from build123d import *

# Parameters (mm, degrees)
SKETCH_W        = 30
SKETCH_H        = 25
PAD_DEPTH       = 30
SKETCH001_W     = 20.784298
SKETCH001_H     = 31.024467
POCKET_DEPTH    = 30.001
POCKET001_DEPTH = 104.489578018
SKETCH003_R     = 1.4
POCKET002_DEPTH = 5
CHAMFER_SIZE    = 2
CHAMFER001_SIZE = 2
CHAMFER002_SIZE = 1


with BuildPart() as part:
    # Sketch → Pad (new body)
    with BuildSketch(Plane.XZ):
        with Locations((0, 12.5)):
            Rectangle(SKETCH_W, SKETCH_H)
    extrude(amount=PAD_DEPTH)

    # Sketch001 (on Face2 of Pad) → Pocket (cut, through all)
    with BuildSketch(Plane(origin=(15, 0, 0), x_dir=(0, 0, 1), z_dir=(1, 0, 0))):
        with Locations((16.392149, 19.5122335)):
            Rectangle(SKETCH001_W, SKETCH001_H)
    extrude(amount=-POCKET_DEPTH, mode=Mode.SUBTRACT)

    # Sketch002 (on Face8 of Pocket) → Pocket001 (cut, through all)
    with BuildSketch(Plane(origin=(0, 0, 6), x_dir=(-1, 0, 0), z_dir=(0, 0, 1))):
        Polygon((-12.1547078033, 18.0000041944), (-7.1547078033, 18.0000041944), (-6, 20), (-7.1546932734, 22.0000041944), (-12.1547078033, 22.0000041944), (-13.3094083417, 20.0000041944), align=None)
    pocket001 = extrude(amount=-POCKET001_DEPTH, mode=Mode.SUBTRACT)

    # Mirrored: Pocket001 across Sketch002 V_Axis
    add(pocket001.mirror(Plane(origin=(0, 0, 6), x_dir=(0, 0, 1), z_dir=(-1, 0, 0))), mode=Mode.SUBTRACT)

    # Sketch003 (on Face4 of Pocket001) → Pocket002 (cut)
    with BuildSketch(Plane.XZ.offset(4)):
        with Locations((0, 20)):
            Circle(SKETCH003_R)
        with Locations((5, 11.3397459621)):
            Circle(SKETCH003_R)
        with Locations((-5, 11.3397459621)):
            Circle(SKETCH003_R)
    extrude(amount=-POCKET002_DEPTH, mode=Mode.SUBTRACT)

    # Chamfer
    chamfer_edges = [part.edges().sort_by_distance(p)[0] for p in [
        (-15, -2, 25),
        (15, -2, 25),
    ]]
    chamfer(chamfer_edges, length=CHAMFER_SIZE)

    # Chamfer001
    chamfer001_edges = [part.edges().sort_by_distance(p)[0] for p in [
        (15, -30, 3),
        (-15, -30, 3),
    ]]
    chamfer(chamfer001_edges, length=CHAMFER001_SIZE)

    # Chamfer002
    chamfer002_edges = [part.edges().sort_by_distance(p)[0] for p in [
        (0, 0, 0),
    ]]
    chamfer(chamfer002_edges, length=CHAMFER002_SIZE)


solid = part.part
Model file for the job. Use its own axes, mm. A direction names the side the tool comes from. Give positions to 0.01 mm unless a question says otherwise; leave off trailing zeros. Order: outer loops, then holes, each group sorted by start corner. A loop starts at its lowest first (then second) coordinate and runs counter-clockwise, first axis right, second up. Notation, with made-up numbers: (88, 60.25) - (120, 60.25) arc R8 ccw to (120, 74.25) - close; hole circle Ø9 at (-19, 17). An arc over 180 degrees is marked (long way). One line per item, written item: value.
Item 1: Tool access for faces 1 (the flat face through (0, -17, 6)), 2 (the flat face through (10, -18, 3)), 3 (the flat face through (-14, -29, 3)): list every direction of +Z, -Z, +X, -X, +Y, -Y with a clear straight run to the whole face (end or side of a thin tool).
Response values:
face 1: +Z, +X, -X, -Y
face 2: +Z, -Z
face 3: +Z, -Z, -X, -Y
Item 2: Wall check: line 1 (Z direction, x = -5, y = -2.2); line 2 (Z direction, x = 0, y = -1.8); line 3 (Z direction, x = 12.25, y = -7.75). Give the ranges that are in metal, low to high.
Response values:
line 1: 0 to 9.94, 12.74 to 25
line 2: 0 to 18.6, 21.4 to 25
line 3: 0 to 6
Item 3: Slice it at A-A (z = 20). List the corners of the cut face in (x, y).
Response values:
outline: (-15, -4) - (-1.4, -4) - (-1.4, 0) - (-15, 0) - close; (1.4, -4) - (15, -4) - (15, 0) - (1.4, 0) - close
Item 4: Slice it at B-B (x = -5). List the corners of the cut face in (y, z), then the cut area to 3 significant figures.
Response values:
outline: (-30, 0) - (-1, 0) - (0, 1) - (0, 9.94) - (-4, 9.94) - (-4, 6) - (-30, 6) - close; (-4, 12.74) - (0, 12.74) - (0, 25) - (-4, 25) - close
area: 244 mm2
Item 5: Two-plate mould, pull along Z, no slides. Class faces 4 (the flat face through (6.57, -20.99, 3.04)), 5 (the cylindrical face through (-0.303, -2.028, 18.633)), 6 (the flat face through (-0.2, -0.5, 0.5)): released by +Z, released by -Z, zero draft, split by the parting line, or undercut.
Response values:
face 4: zero draft
face 5: undercut
face 6: released by -Z
Item 6: Slice it at D-D (y = -6.5). List the corners of the cut face in (x, z).
Response values:
outline: (-15, 0) - (15, 0) - (15, 6) - (-15, 6) - close
Item 7: Slice it at C-C (z = 3.25). List the corners of the cut face in (x, y).
Response values:
outline: (-15, -28) - (-13, -30) - (13, -30) - (15, -28) - (15, 0) - (-15, 0) - close; hole (-13.31, -20) - (-12.15, -22) - (-7.15, -22) - (-6, -20) - (-7.15, -18) - (-12.15, -18) - close; hole (6, -20) - (7.15, -22) - (12.15, -22) - (13.31, -20) - (12.15, -18) - (7.15, -18) - close
Item 8: Pin check, flat tips, straight feed: pin 1 Ø4.5 at (x, z) = (0, 20) entering from -Y; pin 2 Ø3 at (x, y) = (1.5, -24.5) entering from +Z. Stop position of each tip, or through.
Response values:
pin 1: y = -4
pin 2: z = 6
